```python
from build123d import *

# Parameters (mm, degrees)
REVOLVE1_ANGLE      = 180
SKETCH2_W           = 15
SKETCH2_H           = 5
BOSS_EXTRUDE1_DEPTH = 10
FILLET2_R           = 2
FILLET3_R           = 2
FILLET4_R           = 2
FILLET5_R           = 2
FILLET6_R           = 2


with BuildPart() as part:
    # Sketch1 → Revolve1 (revolve)
    with BuildSketch(Plane.XY):
        with BuildLine():
            Line((61, 170), (61, 0))
            Line((61, 0), (58, 0))
            Line((58, 0), (58, 170))
            ThreePointArc((58, 170), (41.873834296, 218.154039035), (0, 246.884627213))
            Line((0, 246.884627213), (0, 250))
            ThreePointArc((0, 250), (44.010282534, 220.301590432), (61, 170))
        make_face()
    revolve(axis=Axis((0, 0, 0), (0, 1, 0)), revolution_arc=REVOLVE1_ANGLE)

    # Sketch2 → Boss-Extrude1 (add)
    with BuildSketch(Plane.XY):
        with Locations((50.5, 167.5)):
            Rectangle(SKETCH2_W, SKETCH2_H)
        with Locations((-50.5, 167.5)):
            Rectangle(SKETCH2_W, SKETCH2_H)
    extrude(amount=-BOSS_EXTRUDE1_DEPTH)

    # Fillet2
    # the kernel refuses this fillet: 2 mm, written as the material it adds along each edge
    with BuildSketch(Plane(origin=(0, 170, 0), x_dir=(1, 0, 0), z_dir=(0, 0, 1))) as fillet2_piece_1_section:
        with BuildLine():
            CenterArc((55.974341272, 2), FILLET2_R, 270, 91.470056164)
            Line((55.974341272, 0), (58, 0))
            ThreePointArc((58, 0), (57.993420482, 1.025738909), (57.97368301, 2.051309011))
        make_face()
    fillet2_piece_1 = revolve(axis=Axis((0, 170, 0), (0, 1, 0)), revolution_arc=14.994639912, mode=Mode.PRIVATE)
    fillet2_piece_1 = split(fillet2_piece_1, bisect_by=Plane(origin=(57.246854663, 170.465829225, -10), z_dir=(0, 0, 1)), keep=Keep.TOP, mode=Mode.PRIVATE)
    add(fillet2_piece_1)
    with BuildSketch(Plane(origin=(0, 170, 0), x_dir=(-0.9659500348920197, 0, -0.2587286804590979), z_dir=(0.2587286804590979, 0, -0.9659500348920197))) as fillet2_piece_2_section:
        with BuildLine():
            CenterArc((55.974341272, 2), FILLET2_R, 270, 91.470056164)
            Line((55.974341272, 0), (58, 0))
            ThreePointArc((58, 0), (57.993420482, 1.025738909), (57.97368301, 2.051309011))
        make_face()
    fillet2_piece_2 = revolve(axis=Axis((0, 170, 0), (0, 1, 0)), revolution_arc=14.994639912, mode=Mode.PRIVATE)
    fillet2_piece_2 = split(fillet2_piece_2, bisect_by=Plane(origin=(-57.246854909, 170.465829269, -10), z_dir=(0, 0, 1)), keep=Keep.TOP, mode=Mode.PRIVATE)
    add(fillet2_piece_2)
    # the kernel refuses this fillet: 2 mm, written as the material it takes off along each edge
    with BuildSketch(Plane(origin=(43, 170, 5), x_dir=(0, -1, 0), z_dir=(0, 0, -1)), Plane(origin=(-43, 170, 5), x_dir=(-1, 0, 0), z_dir=(0, 0, -1))) as fillet2_2_piece_1:
        with BuildLine():
            CenterArc((FILLET2_R, -FILLET2_R), FILLET2_R, 90, 90)
            Line((0, -FILLET2_R), (0, 0))
            Line((0, 0), (FILLET2_R, 0))
        make_face()
    extrude(amount=20, mode=Mode.SUBTRACT)

    # Fillet3
    fillet3_edges = [part.edges().sort_by_distance(p)[0] for p in [
        (57.782448853, 165, -5.01882502),
    ]]
    fillet(fillet3_edges, radius=FILLET3_R)

    # Fillet4
    fillet4_edges = [part.edges().sort_by_distance(p)[0] for p in [
        (-57.782448853, 165, -5.01882502),
    ]]
    fillet(fillet4_edges, radius=FILLET4_R)

    # Fillet5
    fillet5_edges = [part.edges().sort_by_distance(p)[0] for p in [
        (-43, 165, -5),
    ]]
    fillet(fillet5_edges, radius=FILLET5_R)

    # Fillet6
    fillet6_edges = [part.edges().sort_by_distance(p)[0] for p in [
        (43, 165, -5),
    ]]
    fillet(fillet6_edges, radius=FILLET6_R)


solid = part.part
```
Could you check a few things on this model? Use its own coordinates, in mm. A direction names the side the tool comes from. Round coordinates to 2 decimals unless told otherwise and drop trailing zeros. Loops run counter-clockwise (first coordinate to the right, second up) from the corner with the lowest first, then second, coordinate; pieces in that order, holes last.
Q1. Thinking about a two-plate mould opening in Y: for faces 1 (the flat face through (-51, 170, -5)), 2 (the cylindrical face through (1.275, 86.19, -57.986)), 3 (the flat face through (9, 0, -58)), which applies, pulls with the +Y half, pulls with the -Y half, needs draft (parallel to the pull), parting line crosses it, or undercut?
Q2. I want a section at A-A (y = 71). Write out the boundary of the cut face in (x, z).
Q3. Please list where these lines run through material, in increasing order: L1, parallel to X at y = 191.5, z = -23.5; L2, parallel to X at y = 47.5, z = -31.5; L3, parallel to Z at x = 2, y = 95.
Q4. For P1, Ø11, axis at x = -49, z = -2.5, coming from the +Y side; P2, Ø5, axis at y = 72, z = -44.5, coming from the +X side; P3, Ø4, axis at x = -25.5, y = 210.5, coming from the -Z side, each with a flat end and sliding along its axis, tell me the tip position at first contact or that it passes through.
Q5. On a 3-axis mill with a long thin cutter (end or side, diameter ignored), from which of +Z, -Z, +X, -X, +Y, -Y can I reach the whole of each face in a straight line? I mean faces 4 (the flat face through (50, 170, -5)), 5 (the cylindrical face through (1.341, 83.81, -60.985)), 6 (the flat face through (-51, 165, -5)). Say none if no direction works.
Answer below:
1. face 1: undercut
1. face 2: needs draft
1. face 3: pulls with the -Y half
2. outline: (-61, 0) arc R61 ccw to (61, 0) - (58, 0) arc R58 cw to (-58, 0) - close
3. L1: x = -53.21 to -49.79, 49.79 to 53.21
3. L2: x = -52.24 to -48.7, 48.7 to 52.24
3. L3: z = -60.97 to -57.97
4. P1: stops at y = 220.88
4. P2: stops at x = 44.24
4. P3: stops at z = -45.2
5. face 4: +Z
5. face 5: -Z, +Y, -Y
5. face 6: +Z, -Y
